Here's how the part is built. I have some questions about the finished solid (model axes, mm). A direction names the side the tool comes from. Give positions to 0.01 mm unless a question says otherwise; leave off trailing zeros. Loops run counter-clockwise (first coordinate to the right, second up) from the corner with the lowest first, then second, coordinate; pieces in that order, holes last. Notation, with made-up numbers: (-15.75, 17) -> (14.25, 17) arc R27 ccw to (14.25, 42) -> close; hole circle Ø3 at (-20, -38.75). An arc over 180 degrees is marked (long way). Answer in a Markdown table with one row per item. Add a question column.
Item 1: For P1, Ø3, axis at x = 13.5, y = 6.5, coming from the -Z side; P2, Ø4.5, axis at x = -21.5, z = -34.5, coming from the +Y side; P3, Ø6, axis at x = 13.5, z = -39, coming from the -Y side; P4, Ø2.5, axis at x = 72, z = -38, coming from the -Y side, each with a flat end and sliding along its axis, tell me the tip position at first contact or that it passes through.
Item 2: Which directions (+Z, -Z, +X, -X, +Y, -Y) give clear straight access to the entire face, cutting with the end or side of a thin tool? Please do faces 4 (the face through (-69.963, 1.479, 38.689)), 5 (the face through (-24.5, 6, -38.5)), 6 (the face through (70.09, 1.48, -37.01)).
Item 3: If we section it at C-C (z = 19): Write out the boundary of the cut face in (x, y), then the cut area to 3 significant figures.
Item 4: If we section it at D-D (x = -21.5): Write out the boundary of the cut face in (y, z), then the cut area to 3 significant figures.
Item 5: If we section it at B-B (x = 72): Write out the boundary of the cut face in (y, z), then the cut area to 3 significant figures.
Item 6: If we section it at A-A (y = 5): Give the number of separate pieces and of enclosed holes in the cut face, then the cut area to 3 significant figures.
Item 7: If I drill on line 1 (X direction, y = 1.25, z = -38); line 2 (X direction, y = 6.75, z = 19); line 3 (X direction, y = 5.7, z = -34.5), over which ranges is the centre line in solid material (lowest first)?
Item 8: We'd pull the mould along X, two halves only. Please class faces 1 (the face through (-1, 0, -1)), 2 (the face through (63, 3, -39)), 3 (the face through (-80, 1, 1)): released by +X, released by -X, zero draft, split by the parting line, or undercut.
```python
from build123d import *

# Parameters (mm, degrees)
SK_PLATE_W         = 160
SK_PLATE_H         = 90
EX_PLATE_DEPTH     = 3
SK_STANDOFFS_R     = 3
SK_STANDOFFS_R_2   = 5
EX_STANDOFFS_DEPTH = 6
SK_INSERTS_R       = 1.8
SK_INSERTS_R_2     = 2.8
CUT_INSERTS_DEPTH  = 6
SK_PANHOLES_R      = 2.15
CUT_PANHOLES_DEPTH = 3


with BuildPart() as part:
    # SK_Plate → EX_Plate (new body)
    with BuildSketch(Plane(origin=(0, 0, 0), x_dir=(1, 0, 0), z_dir=(0, 1, 0))):
        Rectangle(SK_PLATE_W, SK_PLATE_H)
    extrude(amount=EX_PLATE_DEPTH)

    # SK_Standoffs → EX_Standoffs (add)
    with BuildSketch(Plane(origin=(0, 3, 0), x_dir=(1, 0, 0), z_dir=(0, 1, 0))):
        with Locations(Location((62.5, 39, 0), (0, 0, 270))):
            Circle(SK_STANDOFFS_R)
        with Locations(Location((13.5, 39, 0), (0, 0, 270))):
            Circle(SK_STANDOFFS_R)
        with Locations(Location((62.5, -19, 0), (0, 0, 270))):
            Circle(SK_STANDOFFS_R)
        with Locations(Location((13.5, -19, 0), (0, 0, 270))):
            Circle(SK_STANDOFFS_R)
        with Locations(Location((-21.5, -34.5, 0), (0, 0, 270))):
            Circle(SK_STANDOFFS_R_2)
        with Locations(Location((-68.5, -34.5, 0), (0, 0, 270))):
            Circle(SK_STANDOFFS_R_2)
        with Locations(Location((-21.5, 34.5, 0), (0, 0, 270))):
            Circle(SK_STANDOFFS_R_2)
        with Locations(Location((-68.5, 34.5, 0), (0, 0, 270))):
            Circle(SK_STANDOFFS_R_2)
    extrude(amount=EX_STANDOFFS_DEPTH)

    # SK_Inserts → CUT_Inserts (cut)
    with BuildSketch(Plane(origin=(0, 9, 0), x_dir=(1, 0, 0), z_dir=(0, 1, 0))):
        with Locations(Location((62.5, 39, 0), (0, 0, 270))):
            Circle(SK_INSERTS_R)
        with Locations(Location((13.5, 39, 0), (0, 0, 270))):
            Circle(SK_INSERTS_R)
        with Locations(Location((62.5, -19, 0), (0, 0, 270))):
            Circle(SK_INSERTS_R)
        with Locations(Location((13.5, -19, 0), (0, 0, 270))):
            Circle(SK_INSERTS_R)
        with Locations(Location((-21.5, -34.5, 0), (0, 0, 270))):
            Circle(SK_INSERTS_R_2)
        with Locations(Location((-68.5, -34.5, 0), (0, 0, 270))):
            Circle(SK_INSERTS_R_2)
        with Locations(Location((-21.5, 34.5, 0), (0, 0, 270))):
            Circle(SK_INSERTS_R_2)
        with Locations(Location((-68.5, 34.5, 0), (0, 0, 270))):
            Circle(SK_INSERTS_R_2)
    extrude(amount=-CUT_INSERTS_DEPTH, mode=Mode.SUBTRACT)

    # SK_PanHoles → CUT_PanHoles (cut)
    with BuildSketch(Plane(origin=(0, 0, 0), x_dir=(1, 0, 0), z_dir=(0, 1, 0))):
        with Locations(Location((72, -38, 0), (0, 0, 270))):
            Circle(SK_PANHOLES_R)
        with Locations(Location((-72, -38, 0), (0, 0, 123.831741561))):
            Circle(SK_PANHOLES_R)
        with Locations(Location((72, 38, 0), (0, 0, 270))):
            Circle(SK_PANHOLES_R)
        with Locations(Location((-72, 38, 0), (0, 0, 33.831741561))):
            Circle(SK_PANHOLES_R)
    extrude(amount=CUT_PANHOLES_DEPTH, mode=Mode.SUBTRACT)


solid = part.part
```
Recorded:
| question | item | result |
|---|---|---|
| 1 | P1 | stops at z = -42 |
| 1 | P2 | stops at y = 3 |
| 1 | P3 | stops at y = 0 |
| 1 | P4 | passes through |
| 2 | face 4 | -Y |
| 2 | face 5 | +Y |
| 2 | face 6 | +Y, -Y |
| 3 | outline | (-80, 0) -> (80, 0) -> (80, 3) -> (65.5, 3) -> (65.5, 9) -> (64.3, 9) -> (64.3, 3) -> (60.7, 3) -> (60.7, 9) -> (59.5, 9) -> (59.5, 3) -> (16.5, 3) -> (16.5, 9) -> (15.3, 9) -> (15.3, 3) -> (11.7, 3) -> (11.7, 9) -> (10.5, 9) -> (10.5, 3) -> (-80, 3) -> close |
| 3 | area | 509 mm^2 |
| 4 | outline | (0, -45) -> (3, -45) -> (3, -39.5) -> (9, -39.5) -> (9, -37.3) -> (3, -37.3) -> (3, -31.7) -> (9, -31.7) -> (9, -29.5) -> (3, -29.5) -> (3, 29.5) -> (9, 29.5) -> (9, 31.7) -> (3, 31.7) -> (3, 37.3) -> (9, 37.3) -> (9, 39.5) -> (3, 39.5) -> (3, 45) -> (0, 45) -> close |
| 4 | area | 323 mm^2 |
| 5 | outline | (0, -45) -> (3, -45) -> (3, -40.15) -> (0, -40.15) -> close; (0, -35.85) -> (3, -35.85) -> (3, 35.85) -> (0, 35.85) -> close; (0, 40.15) -> (3, 40.15) -> (3, 45) -> (0, 45) -> close |
| 5 | area | 244 mm^2 |
| 6 | separate pieces | 8 |
| 6 | enclosed holes | 8 |
| 6 | area | 288 mm^2 |
| 7 | line 1 | x = -80 to -74.15, -69.85 to 69.85, 74.15 to 80 |
| 7 | line 2 | x = 10.5 to 11.7, 15.3 to 16.5, 59.5 to 60.7, 64.3 to 65.5 |
| 7 | line 3 | x = -73.5 to -71.3, -65.7 to -63.5, -26.5 to -24.3, -18.7 to -16.5 |
| 8 | face 1 | zero draft |
| 8 | face 2 | undercut |
| 8 | face 3 | released by -X |
